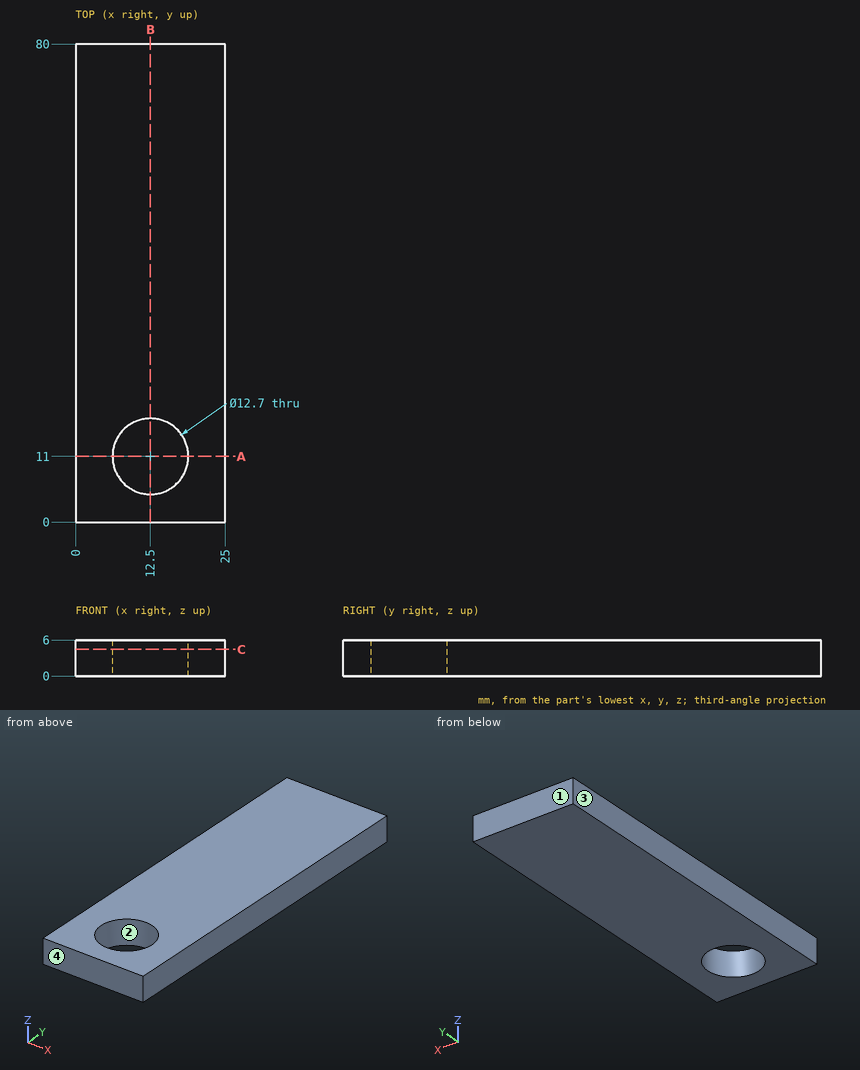
Geometry: see drawing. Coordinates: mm, zero at the bounding-box minimum. Coordinates: 2 decimals unless noted, no trailing zeros. Loops run counter-clockwise (first coordinate to the right, second up) from the corner with the lowest first, then second, coordinate; pieces in that order, holes last.
Q1. Draft query along Y for the marked faces 1, 2, 3 and 4. Return one class per face: +Y half, -Y half, draft (parallel to the pull), parting line (faces both ways), or undercut.
Q2. Cut plane A-A (y = 11). Output: boundary loops of the cut face in (x, z), then the cut area to 3 significant figures.
Q3. Cut plane B-B (x = 12.5). Output: boundary loops of the cut face in (y, z), then the cut area to 3 significant figures.
Q4. Cut plane C-C (z = 4.45). Output: boundary loops of the cut face in (x, y), then the cut area to 3 significant figures.
Q5. Material intervals for line 1 (Y direction, x = 12.5, z = 2.95); line 2 (Y direction, x = 7.5, z = 4.6); line 3 (X direction, y = 14, z = 5.4), sorted ascending.
Working result:
1. face 1: +Y half
1. face 2: undercut
1. face 3: draft
1. face 4: -Y half
2. outline: (0, 0) - (6.15, 0) - (6.15, 6) - (0, 6) - close; (18.85, 0) - (25, 0) - (25, 6) - (18.85, 6) - close
2. area: 73.8 mm2
3. outline: (0, 0) - (4.65, 0) - (4.65, 6) - (0, 6) - close; (17.35, 0) - (80, 0) - (80, 6) - (17.35, 6) - close
3. area: 404 mm2
4. outline: (0, 0) - (25, 0) - (25, 80) - (0, 80) - close; hole circle Ø12.7 at (12.5, 11)
4. area: 1,870 mm2
5. line 1: y = 0 to 4.65, 17.35 to 80
5. line 2: y = 0 to 7.09, 14.91 to 80
5. line 3: x = 0 to 6.9, 18.1 to 25
